Could you check a few things on this model? Use its own coordinates, in mm. A direction names the side the tool comes from. Round coordinates to 2 decimals unless told otherwise and drop trailing zeros. Order: outer loops, then holes, each group sorted by start corner. A loop starts at its lowest first (then second) coordinate and runs counter-clockwise, first axis right, second up. Notation, with made-up numbers: (14, 38.25) - (63, 38.25) arc R21 cw to (63, 52.25) - close; hole circle Ø9 at (33, 39.5). An arc over 180 degrees is marked (long way). Use one line per item in the form item = value.
from build123d import *

# Parameters (mm, degrees)
BOSS_EXTRUDE1_DEPTH = 19.999999553
SKETCH2_W           = 29.999999329
SKETCH2_H           = 7.099999115
CUT_EXTRUDE1_DEPTH  = 55.335457568
SKETCH3_W           = 7.599998266
SKETCH3_H           = 7.099999115
CUT_EXTRUDE2_DEPTH  = 55.335457568
SKETCH4_W           = 1.599997282
SKETCH4_H           = 3.620889969
CUT_EXTRUDE3_DEPTH  = 55.335457568
BOSS_EXTRUDE2_REACH = 56.335
SKETCH6_W           = 3.500001505
SKETCH6_H           = 7.10000284
SKETCH7_R           = 4
BOSS_EXTRUDE3_DEPTH = 7
MOVE_FACE2_BY       = 6


with BuildPart() as part:
    # Sketch1 → Boss-Extrude1 (new body)
    with BuildSketch(Plane(origin=(10, 0, 0), x_dir=(0, 0, -1), z_dir=(1, 0, 0))):
        Polygon((0, 29.379108921), (-35.59999913, 29.379108921), (-41.0999991, 7.000000216), (-41.0999991, -17.7208893), (0, -17.7208893), align=None)
    extrude(amount=-BOSS_EXTRUDE1_DEPTH)

    # Sketch2 → Cut-Extrude1 (cut, through all)
    with BuildSketch(Plane(origin=(10, 0, 0), x_dir=(0, 0, -1), z_dir=(1, 0, 0))):
        with Locations((-14.999999665, -14.170889742)):
            Rectangle(SKETCH2_W, SKETCH2_H)
    extrude(amount=-CUT_EXTRUDE1_DEPTH, mode=Mode.SUBTRACT)

    # Sketch3 → Cut-Extrude2 (cut, through all)
    with BuildSketch(Plane(origin=(10, 0, 0), x_dir=(0, 0, -1), z_dir=(1, 0, 0))):
        with Locations((-37.299999967, -14.170889742)):
            Rectangle(SKETCH3_W, SKETCH3_H)
    extrude(amount=-CUT_EXTRUDE2_DEPTH, mode=Mode.SUBTRACT)

    # Sketch4 → Cut-Extrude3 (cut, through all)
    with BuildSketch(Plane(origin=(10, 0, 0), x_dir=(0, 0, -1), z_dir=(1, 0, 0))):
        with Locations((-40.300000459, -8.810445201)):
            Rectangle(SKETCH4_W, SKETCH4_H)
    extrude(amount=-CUT_EXTRUDE3_DEPTH, mode=Mode.SUBTRACT)

    # Boss-Extrude2: up to this plane
    boss_extrude2_end = Plane(origin=(-9.873244788, 0, -0.038787862), z_dir=(-0.9999922832070416, 0, -0.003928552706520363))
    # Sketch6 → Boss-Extrude2 (add, up to the surface)
    with BuildSketch(Plane(origin=(10, 0, 0), x_dir=(0, 0, -1), z_dir=(1, 0, 0)), mode=Mode.PRIVATE) as boss_extrude2_sk1:
        with Locations((-31.750000082, 32.929110341)):
            Rectangle(SKETCH6_W, SKETCH6_H)
    boss_extrude2_tool1 = split(extrude(boss_extrude2_sk1.sketch, amount=-BOSS_EXTRUDE2_REACH, mode=Mode.PRIVATE), bisect_by=boss_extrude2_end, keep=Keep.BOTH, mode=Mode.PRIVATE)
    add(boss_extrude2_tool1.solids().sort_by_distance((10, 32.92911, 31.75))[0])

    # Sketch7 → Boss-Extrude3 (add)
    with BuildSketch(Plane.XY.offset(41.0999991)):
        Circle(SKETCH7_R)
    extrude(amount=BOSS_EXTRUDE3_DEPTH)

    # Move Face2: a face moved outward by 6.0
    extrude(part.faces().sort_by_distance((0, 0, 48.0999991))[0], amount=MOVE_FACE2_BY, dir=(0, 0, 1))


solid = part.part
Item 1: For faces 1 (the face through (0, -14, 30)), 2 (the face through (-0.867, -3.905, 47.509)), 3 (the face through (0, -7, 40)), 4 (the face through (0, 33, 33.5)), 5 (the face through (0, 29.379, 12)), which set-ups out of +Z, -Z, +X, -X, +Y, -Y let a thin tool reach every point of the face, with its end or its side?
Found:
face_1 = -Z, +X, -X, -Y
face_2 = +Z
face_3 = +Z, +X, -X, -Y
face_4 = +Z, +X, -X, +Y
face_5 = -Z, +X, -X, +Y
Item 2: Imagine slicing it at B-B on y = 0. Please give me the cut outline in (x, z), plus the area to 3 significant figures.
Found:
outline = (-10, 0) - (10, 0) - (10, 41.1) - (4, 41.1) - (4, 54.1) - (-4, 54.1) - (-4, 41.1) - (-10, 41.1) - close
area = 926 mm2
Item 3: Imagine slicing it at C-C on x = -8.5. Please give me the cut outline in (y, z), plus the area to 3 significant figures.
Found:
outline = (-17.72, 30) - (-10.62, 30) - (-10.62, 0) - (29.38, 0) - (29.38, 30) - (36.48, 30) - (36.48, 33.5) - (29.38, 33.5) - (29.38, 35.6) - (7, 41.1) - (-7, 41.1) - (-7, 39.5) - (-10.62, 39.5) - (-10.62, 33.5) - (-17.72, 33.5) - close
area = 1,630 mm2
Item 4: I need wall thicknesses on L1, parallel to X at y = 8.5, z = 17; L2, parallel to Z at x = -4.5, y = 5.5; L3, parallel to Z at x = 9, y = 32. Which ranges of each line are inside material? Lowest first, please.
Found:
L1 = -10 to 10
L2 = 0 to 41.1
L3 = 30 to 33.5
Item 5: Imagine slicing it at A-A on x = 0. Please give me the cut outline in (y, z), plus the area to 3 significant figures.
Found:
outline = (-17.72, 30) - (-10.62, 30) - (-10.62, 0) - (29.38, 0) - (29.38, 30) - (36.48, 30) - (36.48, 33.5) - (29.38, 33.5) - (29.38, 35.6) - (7, 41.1) - (4, 41.1) - (4, 54.1) - (-4, 54.1) - (-4, 41.1) - (-7, 41.1) - (-7, 39.5) - (-10.62, 39.5) - (-10.62, 33.5) - (-17.72, 33.5) - close
area = 1,730 mm2
Item 6: Will these pins go through, and if not, where does the flat tip stop? P1, Ø10, axis at x = 4, z = 12.5, coming from the -Y side; P2, Ø3.5, axis at x = 2.5, y = 34, coming from the -Z side; P3, Ø1, axis at x = 0, z = 34.5, coming from the +Y side.
Found:
P1 = -10.62
P2 = 30
P3 = 29.38
Item 7: Imagine slicing it at D-D on z = 11.5. Please give me the cut outline in (x, y), plus the area to 3 significant figures.
Found:
outline = (-10, -10.62) - (10, -10.62) - (10, 29.38) - (-10, 29.38) - close
area = 800 mm2
